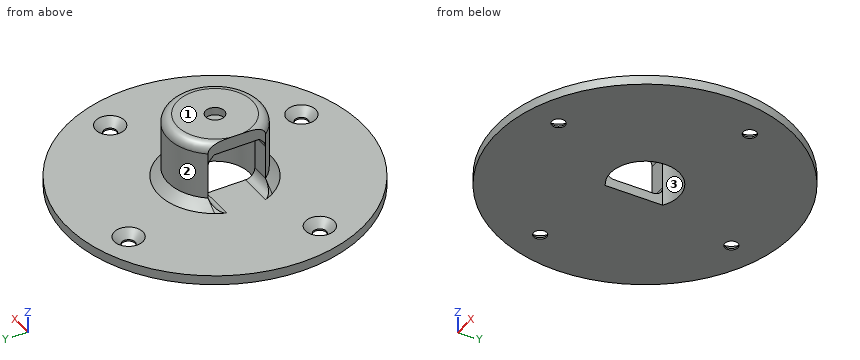
Autodesk Inventor part; units mm, degrees
ref_plane "YZ Plane" through (0, 0, 0) normal (1, 0, 0) x (0, 1, 0)
ref_plane "XZ Plane" through (0, 0, 0) normal (0, 1, 0) x (-1, 0, 0)
ref_plane "XY Plane" through (0, 0, 0) normal (0, 0, 1) x (1, 0, 0)
sketch "Skizze1" plane through (0, 0, 0) normal (0, 0, 1) x (1, 0, 0)
  circle A0 centre (-35.2385, -12.8258) radius 2.1
  circle A1 centre (-12.8258, 35.2385) radius 2.1
  circle A2 centre (12.8258, -35.2385) radius 2.1
  circle A3 centre (35.2385, 12.8258) radius 2.1
  circle A4 centre (0, 0) radius 25
  circle A5 centre (0, 0) radius 45
  circle A6 centre (0, 0) radius 47.5
  circle A7 centre (0, 0) radius 8.4675
  point P0 (0, 0)
extrude "Extrusion1" add sketch "Skizze1" along normal blind 3 contours A4 | A5 | A6 | A7
sketch "Skizze2" plane through (0, 0, 3) normal (0, 0, 1) x (1, 0, 0)
  circle A0 centre (0, 0) radius 15
  dimension "d2" = 30
extrude "Extrusion2" add sketch "Skizze2" along normal blind 21
sketch "Skizze3" plane through (0, 0, 24) normal (0, 0, 1) x (1, 0, 0)
  circle A0 centre (0, 0) radius 3
  dimension "d7" = 6
extrude "Extrusion3" cut sketch "Skizze3" against normal blind 2.5
sketch "Skizze4" plane through (0, 0, 0) normal (0, 0, -1) x (-1, 0, 0)
  circle A0 centre (0, 0) radius 15
  circle A1 centre (0, 0) radius 11
  dimension "d8" = 4
extrude "Extrusion4" cut sketch "Skizze4" against normal blind 20 contours A1
sketch "Skizze5" plane through (0, 0, 0) normal (0, 0, -1) x (-1, 0, 0)
  circle A0 centre (0, 0) radius 11
  circle A1 centre (-35.2385, 12.8258) radius 2.1
  circle A2 centre (-12.8258, -35.2385) radius 2.1
  circle A3 centre (12.8258, 35.2385) radius 2.1
  circle A4 centre (35.2385, -12.8258) radius 2.1
  circle A5 centre (0, 0) radius 47.5
  line L0 (6, -9.2195) -> (6, 9.2195)
  dimension "d11" = 6
extrude "Extrusion5" add sketch "Skizze5" against normal up to surface (20 mm away) contours A0 L0 picked at (7.6667, 0)
sketch "Skizze6" plane through (-6, -9.2195, 0) normal (1, 0, 0) x (0, 0, -1)
  line L0 (-20, 0) -> (-20, 18.4391)
  line L1 (0, 0) -> (-20, 0)
  line L2 (0, 18.4391) -> (0, 0)
  line L3 (-20, 18.4391) -> (0, 18.4391)
  line L4 (-3, -5.7805) -> (-3, 24.2195)
  line L5 (-3, 19.9453) -> (-3, 24.1453)
  line L6 (-3, -28.1189) -> (-3, -23.9189)
  line L7 (-3, 42.358) -> (-3, 46.558)
  line L8 (-3, -5.7062) -> (-3, -1.5062)
  line L9 (-3, 56.7195) -> (-3, -38.2805)
  line L10 (-3, 0) -> (-20, 0)
  line L11 (-20, 0) -> (-20, 18.4391)
  line L12 (-20, 18.4391) -> (-3, 18.4391)
  line L13 (-3, 18.4391) -> (-3, 0)
  point P0 (0, 9.2195)
extrude "Extrusion6" cut sketch "Skizze6" against normal blind 20 contours L0 L3 L4 L1
sketch "Skizze7" plane through (0, 0, 20) normal (0, 0, -1) x (-1, 0, 0)
  arc A0 (6, 9.2195) -> (6, -9.2195) centre (0, 0) ccw
  line L0 (6, -9.2195) -> (11.8322, -9.2195)
  arc A1 (11.8322, -9.2195) -> (11.8322, 9.2195) centre (0, 0) ccw
  line L1 (6, 9.2195) -> (11.8322, 9.2195)
  line L2 (11.8322, 9.2195) -> (11.8322, -9.2195)
extrude "Extrusion7" cut sketch "Skizze7" against normal blind 20 contours A1 L2
chamfer "Fase1" distance 3 angle 45 1 edges at (15, 0, 3)
chamfer "Fase2" distance 2.5 angle 45 4 edges at (-14.9258, 35.2385, 3) (33.1385, 12.8258, 3) (10.7258, -35.2385, 3) (-37.3385, -12.8258, 3)
fillet "Rundung1" radius 3 2 edges at (-10.7298, 9.2195, 3) (-10.7298, -9.2195, 3)
chamfer "Fase3" distance 2 angle 45 2 edges at (-8.9161, 9.2195, 20) (-8.9161, -9.2195, 20)
fillet "Rundung2" radius 3 2 edges at (-8.9161, 9.2195, 18) (-8.9161, -9.2195, 18)
fillet "Rundung3" radius 3 1 edges at (15, 0, 24)
properties part number "OberArmMagnet" material "ABS-Kunststoff"
Work out the finished part from the listing and answer in its coordinate system (mm). Face numbers are marked on the shaded views. Give positions to 0.01 mm unless a question says otherwise; leave off trailing zeros. Order: outer loops, then holes, each group sorted by start corner. A loop starts at its lowest first (then second) coordinate and runs counter-clockwise, first axis right, second up. Notation, with made-up numbers: (2, -1) - (57, -1) arc R6 ccw to (57, 8) - close; hole circle Ø3 at (62.5, 17). An arc over 180 degrees is marked (long way). One line per item, written item: value. Start each with the question number.
1. For a pull along Y with two mould halves and no side action, classify the marked faces 1, 2 and 3 as released by +Y, released by -Y, zero draft, split by the parting line, or undercut.
2. Section C-C, the plane z = 14 is taken. Write down the section's boundary in (x, y), then the cut area to 3 significant figures.
3. Consider line 1 (Z direction, x = 10.5, y = 0.5); line 2 (Y direction, x = 0, z = 22.8); line 3 (Z direction, x = -5.5, y = -37). Determine where each line is inside the solid, lowest interval first.
4. Section B-B, the plane x = 0 is taken. Write down the section's boundary in (y, z).
5. Section A-A, the plane y = 0 is taken. Write down the section's boundary in (x, z).
6. Each of these flat-tipped pins is pushed along its axis until it touches: pin 1 Ø1 at (x, z) = (-17, 4.5) entering from -Y; pin 2 Ø1.7 at (x, z) = (-8, 11) entering from -Y; pin 3 Ø1.7 at (x, z) = (-8, 13) entering from +Y; pin 4 Ø2 at (x, z) = (24.5, 3.5) entering from -Y. Where does it stop, or does it pass through?
7. Section D-D, the plane y = -23 is taken. Write down the section's boundary in (x, z), then the cut area to 3 significant figures.
Filled sheet:
1. face 1: zero draft
1. face 2: split by the parting line
1. face 3: undercut
2. outline: (-11.83, -9.22) arc R15 ccw (long way) to (-11.83, 9.22) - (-6, 9.22) arc R11 cw (long way) to (-6, -9.22) - close
2. area: 244 mm²
3. line 1: 20 to 24
3. line 2: -14.4 to -3, 3 to 14.4
3. line 3: 0 to 3
4. outline: (-47.5, 0) - (-11, 0) - (-11, 20) - (11, 20) - (11, 0) - (47.5, 0) - (47.5, 3) - (18, 3) - (15, 6) - (15, 21) arc R3 ccw to (12, 24) - (3, 24) - (3, 21.5) - (-3, 21.5) - (-3, 24) - (-12, 24) arc R3 ccw to (-15, 21) - (-15, 6) - (-18, 3) - (-47.5, 3) - close
5. outline: (-47.5, 0) - (-6, 0) - (-6, 3) - (-47.5, 3) - close; (-11.83, 20) - (11, 20) - (11, 0) - (47.5, 0) - (47.5, 3) - (18, 3) - (15, 6) - (15, 21) arc R3 ccw to (12, 24) - (3, 24) - (3, 21.5) - (-3, 21.5) - (-3, 24) - (-11.83, 24) - close
6. pin 1: through
6. pin 2: y = -13.19
6. pin 3: y = 13.19
6. pin 4: y = -41.2
7. outline: (-41.56, 0) - (41.56, 0) - (41.56, 3) - (-41.56, 3) - close
7. area: 249 mm²
